Build history of the part. All positions in model axes, mm. Give positions to 0.01 mm unless a question says otherwise; leave off trailing zeros. Loops run counter-clockwise (first coordinate to the right, second up) from the corner with the lowest first, then second, coordinate; pieces in that order, holes last. Notation, with made-up numbers: (-28.75, -16) - (12.25, -16) arc R10 ccw to (12.25, -11) - close; hole circle Ø7 at (-0.75, -29.75). An arc over 180 degrees is marked (long way). Return JSON: item names as keys, results as strings. Group by question number.
1) Slice it at B-B (z = -52.5). List the corners of the cut face in (x, y), and give its area (3 significant figures).
2) Slice it at A-A (x = 0). List the corners of the cut face in (y, z).
3) Drill centre lines: probe 1 along Z at (x, y) = (8.75, 0); probe 2 along X at (y, z) = (0.5, -13.5); probe 3 along Y at (x, z) = (0, -42). Where is each one in solid material? Low to high. Write a range as from..to.
4) Drop flat-ended pins along their axis: pin 1 (2 mm diameter, centred on y = -6.5, z = -21, fed in from +X); pin 2 (8 mm diameter, centred on x = 7.5, z = 83.5, fed in from -Y); pin 3 (2 mm diameter, centred on y = -8, z = -71.5, fed in from -X). Give the stop position or say it passes through.
5) Mould opens along Y. For faces 1 (the face through (9.119, 0.601, 110.592)), 2 (the face through (-4.5, -7.4, -125)), 3 (the face through (-9.119, 0.601, 110.592)) say: released by +Y, released by -Y, zero draft, split by the parting line, or undercut.
```python
from build123d import *

# Parameters (mm, degrees)
SKETCH1_R           = 10
SKETCH1_R_2         = 8.5
BOSS_EXTRUDE1_DEPTH = 125
SKETCH2_R           = 2
CUT_EXTRUDE1_DEPTH  = 126.797456254


with BuildPart() as part:
    # Sketch1 → Boss-Extrude1 (new body)
    with BuildSketch(Plane.XY):
        Circle(SKETCH1_R)
        Circle(SKETCH1_R_2, mode=Mode.SUBTRACT)
    boss_extrude1 = extrude(amount=BOSS_EXTRUDE1_DEPTH)

    # Sketch2 → Cut-Extrude1 (cut, symmetric)
    with BuildSketch(Plane(origin=(0, 0, 0), x_dir=(0, 0, -1), z_dir=(1, 0, 0))):
        with Locations((-112.5, 0)):
            Circle(SKETCH2_R)
        with Locations((-227.5, 0)):
            Circle(SKETCH2_R)
    cut_extrude1 = extrude(amount=CUT_EXTRUDE1_DEPTH, both=True, mode=Mode.SUBTRACT)

    # Mirror1: Boss-Extrude1, Cut-Extrude1 across plane
    add(boss_extrude1.mirror(Plane.XY))
    add(cut_extrude1.mirror(Plane.XY), mode=Mode.SUBTRACT)


solid = part.part
```
Results:
{
 "1": {"outline": "circle Ø20 at (0, 0); hole circle Ø17 at (0, 0)", "area": "87.2 mm2"},
 "2": {"outline": "(-10, -125) - (-8.5, -125) - (-8.5, 125) - (-10, 125) - close; (8.5, -125) - (10, -125) - (10, 125) - (8.5, 125) - close"},
 "3": {"probe 1": "-125..-114.5, -110.5..110.5, 114.5..125", "probe 2": "-9.99..-8.49, 8.49..9.99", "probe 3": "-10..-8.5, 8.5..10"},
 "4": {"pin 1": "x = 8.35", "pin 2": "y = -9.37", "pin 3": "x = -7.14"},
 "5": {"face 1": "undercut", "face 2": "zero draft", "face 3": "undercut"}
}
